```python
from build123d import *

# Parameters (mm, degrees)
SKETCH1_W           = 40
SKETCH1_H           = 24
BOSS_EXTRUDE1_DEPTH = 1
SKETCH2_W           = 40
SKETCH2_H           = 24
SKETCH2_W_2         = 21
SKETCH2_H_2         = 17.5
SKETCH2_W_3         = 13
SKETCH2_H_3         = 18.5
BOSS_EXTRUDE3_DEPTH = 9
SKETCH3_W           = 1
SKETCH3_H           = 17.5
CUT_EXTRUDE2_DEPTH  = 3
SKETCH4_W           = 10.24
SKETCH4_H           = 11.92
BOSS_EXTRUDE4_DEPTH = 1.21
CUT_EXTRUDE3_DEPTH  = 2
SKETCH8_W           = 4
SKETCH8_H           = 18.5
CUT_EXTRUDE4_DEPTH  = 5
SKETCH11_W          = 24
SKETCH11_H          = 10
CUT_EXTRUDE5_DEPTH  = 2
SKETCH12_W          = 4
SKETCH12_H          = 3
CUT_EXTRUDE6_DEPTH  = 3
BOSS_EXTRUDE5_DEPTH = 3.5
SKETCH14_W          = 1
SKETCH14_H          = 2.25
CUT_EXTRUDE7_DEPTH  = 3
SKETCH15_W          = 38
SKETCH15_H          = 10
CUT_EXTRUDE8_DEPTH  = 0.25
SKETCH16_W          = 38
SKETCH16_H          = 10
CUT_EXTRUDE9_DEPTH  = 0.25
SKETCH17_W          = 18.5
SKETCH17_H          = 4
CUT_EXTRUDE10_DEPTH = 0.5


with BuildPart() as part:
    # Sketch1 → Boss-Extrude1 (new body)
    with BuildSketch(Plane(origin=(0, 0, 0), x_dir=(1, 0, 0), z_dir=(0, 1, 0))):
        with Locations((20, 12)):
            Rectangle(SKETCH1_W, SKETCH1_H)
    extrude(amount=BOSS_EXTRUDE1_DEPTH)

    # Sketch2 → Boss-Extrude3 (add)
    with BuildSketch(Plane(origin=(0, 1, 0), x_dir=(1, 0, 0), z_dir=(0, 1, 0))):
        with Locations((20, 12)):
            Rectangle(SKETCH2_W, SKETCH2_H)
        with Locations((11.5, 12)):
            Rectangle(SKETCH2_W_2, SKETCH2_H_2, mode=Mode.SUBTRACT)
        with Locations((29.5, 12)):
            Rectangle(SKETCH2_W_3, SKETCH2_H_3, mode=Mode.SUBTRACT)
    extrude(amount=BOSS_EXTRUDE3_DEPTH)

    # Sketch3 → Cut-Extrude2 (cut)
    with BuildSketch(Plane(origin=(0, 10, 0), x_dir=(1, 0, 0), z_dir=(0, 1, 0))):
        with Locations((22.5, 12)):
            Rectangle(SKETCH3_W, SKETCH3_H)
    extrude(amount=-CUT_EXTRUDE2_DEPTH, mode=Mode.SUBTRACT)

    # Sketch4 → Boss-Extrude4 (add)
    with BuildSketch(Plane(origin=(0, 1, 0), x_dir=(1, 0, 0), z_dir=(0, 1, 0))):
        with Locations((13.26, 12)):
            Rectangle(SKETCH4_W, SKETCH4_H)
    extrude(amount=BOSS_EXTRUDE4_DEPTH)

    # Sketch5 → Cut-Extrude3 (cut)
    with BuildSketch(Plane(origin=(1, 0, 0), x_dir=(0, 0, -1), z_dir=(1, 0, 0))):
        with BuildLine():
            Line((7.53, 2.25), (7.53, 2.96))
            Line((7.53, 2.96), (7.53, 10))
            Line((7.53, 10), (16.47, 10))
            Line((16.47, 10), (16.47, 2.96))
            Line((16.47, 2.96), (16.47, 2.25))
            ThreePointArc((16.47, 2.25), (16.103883476, 1.366116524), (15.22, 1))
            Line((15.22, 1), (8.78, 1))
            ThreePointArc((8.78, 1), (7.896116524, 1.366116524), (7.53, 2.25))
        make_face()
    extrude(amount=-CUT_EXTRUDE3_DEPTH, mode=Mode.SUBTRACT)

    # Sketch8 → Cut-Extrude4 (cut)
    with BuildSketch(Plane(origin=(0, 10, 0), x_dir=(1, 0, 0), z_dir=(0, 1, 0))):
        with Locations((38, 12)):
            Rectangle(SKETCH8_W, SKETCH8_H)
    extrude(amount=-CUT_EXTRUDE4_DEPTH, mode=Mode.SUBTRACT)

    # Sketch11 → Cut-Extrude5 (cut)
    with BuildSketch(Plane(origin=(40, 0, 0), x_dir=(0, 0, -1), z_dir=(1, 0, 0))):
        with Locations((12, 5)):
            Rectangle(SKETCH11_W, SKETCH11_H)
    extrude(amount=-CUT_EXTRUDE5_DEPTH, mode=Mode.SUBTRACT)

    # Sketch12 → Cut-Extrude6 (cut)
    with BuildSketch(Plane(origin=(0, 10, 0), x_dir=(1, 0, 0), z_dir=(0, 1, 0))):
        with Locations((6, 2.5)):
            Rectangle(SKETCH12_W, SKETCH12_H)
    extrude(amount=-CUT_EXTRUDE6_DEPTH, mode=Mode.SUBTRACT)

    # Sketch13 → Boss-Extrude5 (add)
    with BuildSketch(Plane(origin=(0, 10, 0), x_dir=(1, 0, 0), z_dir=(0, 1, 0))):
        Polygon((1, 16.47), (1, 20.75), (3, 20.75), (3, 15.25), (2, 15.25), (2, 16.25), (0, 16.25), (0, 16.47), align=None)
        Polygon((1, 3.25), (3, 3.25), (3, 8.75), (2, 8.75), (2, 7.75), (0, 7.75), (0, 7.53), (1, 7.53), align=None)
    extrude(amount=-BOSS_EXTRUDE5_DEPTH)

    # Sketch14 → Cut-Extrude7 (cut)
    with BuildSketch(Plane(origin=(0, 10, 0), x_dir=(1, 0, 0), z_dir=(0, 1, 0))):
        with Locations((3.5, 2.125)):
            Rectangle(SKETCH14_W, SKETCH14_H)
    extrude(amount=-CUT_EXTRUDE7_DEPTH, mode=Mode.SUBTRACT)

    # Sketch15 → Cut-Extrude8 (cut)
    with BuildSketch(Plane(origin=(0, 0, -24), x_dir=(-1, 0, 0), z_dir=(0, 0, -1))):
        with Locations((-19, 5)):
            Rectangle(SKETCH15_W, SKETCH15_H)
    extrude(amount=-CUT_EXTRUDE8_DEPTH, mode=Mode.SUBTRACT)

    # Sketch16 → Cut-Extrude9 (cut)
    with BuildSketch(Plane.XY):
        with Locations((19, 5)):
            Rectangle(SKETCH16_W, SKETCH16_H)
    extrude(amount=-CUT_EXTRUDE9_DEPTH, mode=Mode.SUBTRACT)

    # Sketch17 → Cut-Extrude10 (cut)
    with BuildSketch(Plane.ZY.offset(-36)):
        with Locations((-12, 3)):
            Rectangle(SKETCH17_W, SKETCH17_H)
    extrude(amount=-CUT_EXTRUDE10_DEPTH, mode=Mode.SUBTRACT)


solid = part.part
```
Could you check a few things on this model? Use its own coordinates, in mm. A direction names the side the tool comes from. Round coordinates to 2 decimals unless told otherwise and drop trailing zeros. Loops run counter-clockwise (first coordinate to the right, second up) from the corner with the lowest first, then second, coordinate; pieces in that order, holes last. Notation, with made-up numbers: (81, 85.5) -> (128, 85.5) arc R24 cw to (128, 102.5) -> close; hole circle Ø5 at (64, 29). An arc over 180 degrees is marked (long way). Put each result on its own line as item: value.
Q1. I want a section at B-B on z = -9.25. Write out the boundary of the cut face in (x, y).
Checks:
outline: (0, 0) -> (38, 0) -> (38, 5) -> (36.5, 5) -> (36.5, 1) -> (23, 1) -> (23, 7) -> (22, 7) -> (22, 1) -> (18.38, 1) -> (18.38, 2.21) -> (8.14, 2.21) -> (8.14, 1) -> (0, 1) -> close
Q2. Please list where these lines run through material, in increasing order: line 1 (X direction, y = 1.5, z = -17.75); line 2 (X direction, y = 1.75, z = -3.75); line 3 (X direction, y = 4.75, z = -10). Write a range as from..to.
Checks:
line 1: 0..1, 8.14..18.38, 22..23, 36.5..38
line 2: 0..1, 22..23, 36.5..38
line 3: 22..23, 36.5..38
Q3. I want a section at C-C on y = 2.75. Write out the boundary of the cut face in (x, z).
Checks:
outline: (0, -23.75) -> (38, -23.75) -> (38, -0.25) -> (0, -0.25) -> (0, -7.53) -> (1, -7.53) -> (1, -3.25) -> (22, -3.25) -> (22, -20.75) -> (1, -20.75) -> (1, -16.47) -> (0, -16.47) -> close; hole (23, -21.25) -> (36.5, -21.25) -> (36.5, -2.75) -> (23, -2.75) -> close
Q4. For pin 1 Ø1 at (y, z) = (8, -3.5) entering from +X; pin 2 Ø3 at (x, z) = (13.5, -19) entering from -Y; pin 3 Ø0.7 at (x, z) = (4.5, -1.5) entering from +Y; pin 4 Ø3 at (x, z) = (6.5, -13) entering from +Y, each with a flat end and sliding along its axis, tell me the tip position at first contact or that it passes through.
Checks:
pin 1: x = 23
pin 2: y = 0
pin 3: y = 7
pin 4: y = 1
Q5. Which directions (+Z, -Z, +X, -X, +Y, -Y) give clear straight access to the entire face, cutting with the end or side of a thin tool? Please do faces 5 (the flat face through (1, 8, -7.75)), 6 (the flat face through (0.5, 4.3, -7.53)), 7 (the flat face through (8, 9, -2)).
Checks:
face 5: -X, +Y
face 6: -X
face 7: +Y
Q6. Thinking about a two-plate mould opening in Y: for faces 1 (the flat face through (5, 9, -1)), 2 (the flat face through (1, 4, -19)), 3 (the flat face through (37, 5, -12)), 4 (the cylindrical face through (0.507, 1.376, -16.114)), which applies, pulls with the +Y half, pulls with the -Y half, needs draft (parallel to the pull), parting line crosses it, or undercut?
Checks:
face 1: needs draft
face 2: undercut
face 3: pulls with the +Y half
face 4: undercut
Q7. I want a section at D-D on x = 29. Write out the boundary of the cut face in (y, z), and give its area (3 significant figures).
Checks:
outline: (0, -23.75) -> (10, -23.75) -> (10, -21.25) -> (1, -21.25) -> (1, -2.75) -> (10, -2.75) -> (10, -0.25) -> (0, -0.25) -> close
area: 68.5 mm2
Q8. I want a section at A-A on y = 8. Write out the boundary of the cut face in (x, z), and give its area (3 significant figures).
Checks:
outline: (0, -23.75) -> (38, -23.75) -> (38, -21.25) -> (23, -21.25) -> (23, -20.75) -> (3, -20.75) -> (3, -15.25) -> (2, -15.25) -> (2, -16.25) -> (0, -16.25) -> close; (0, -7.75) -> (2, -7.75) -> (2, -8.75) -> (3, -8.75) -> (3, -1) -> (8, -1) -> (8, -3.25) -> (23, -3.25) -> (23, -2.75) -> (38, -2.75) -> (38, -0.25) -> (0, -0.25) -> close
area: 231 mm2
